from build123d import *

# Parameters (mm, degrees)
SKETCH1_W           = 73
SKETCH1_H           = 20
BOSS_EXTRUDE1_DEPTH = 40
CUT_EXTRUDE1_DEPTH  = 20
FILLET1_R           = 20
FILLET2_R           = 20


with BuildPart() as part:
    # Sketch1 → Boss-Extrude1 (new body)
    with BuildSketch(Plane(origin=(0, 0, 0), x_dir=(1, 0, 0), z_dir=(0, 1, 0))):
        Rectangle(SKETCH1_W, SKETCH1_H)
    extrude(amount=BOSS_EXTRUDE1_DEPTH)

    # Sketch2 → Cut-Extrude1 (cut)
    with BuildSketch(Plane.XY.offset(10)):
        with BuildLine():
            Line((-29, 0), (-29, 2.352421437))
            ThreePointArc((-29, 2.352421437), (-29.878679656, 4.473741781), (-32, 5.352421437))
            Line((-32, 5.352421437), (-33, 5.352421437))
            ThreePointArc((-33, 5.352421437), (-33.707106781, 5.645314656), (-34, 6.352421437))
            Line((-34, 6.352421437), (-34, 9.352421437))
            ThreePointArc((-34, 9.352421437), (-33.707106781, 10.059528218), (-33, 10.352421437))
            Line((-33, 10.352421437), (-31, 10.352421437))
            Line((-31, 10.352421437), (-28, 10.352421437))
            ThreePointArc((-28, 10.352421437), (-25.171572875, 11.523994313), (-24, 14.352421437))
            Line((-24, 14.352421437), (-24, 37))
            Line((-24, 37), (24, 37))
            Line((24, 37), (24, 14.352421437))
            ThreePointArc((24, 14.352421437), (25.171572875, 11.523994313), (28, 10.352421437))
            Line((28, 10.352421437), (31, 10.352421437))
            Line((31, 10.352421437), (33, 10.352421437))
            ThreePointArc((33, 10.352421437), (33.707106781, 10.059528218), (34, 9.352421437))
            Line((34, 9.352421437), (34, 6.352421437))
            ThreePointArc((34, 6.352421437), (33.707106781, 5.645314656), (33, 5.352421437))
            Line((33, 5.352421437), (32, 5.352421437))
            ThreePointArc((32, 5.352421437), (29.878679656, 4.473741781), (29, 2.352421437))
            Line((29, 2.352421437), (29, 0))
            Line((29, 0), (-29, 0))
        make_face()
    extrude(amount=-CUT_EXTRUDE1_DEPTH, mode=Mode.SUBTRACT)

    # Fillet1
    fillet1_edges = [part.edges().sort_by_distance(p)[0] for p in [
        (36.5, 40, 0),
        (-36.5, 40, 0),
    ]]
    fillet(fillet1_edges, radius=FILLET1_R)

    # Fillet2
    fillet2_edges = [part.edges().sort_by_distance(p)[0] for p in [
        (-24, 37, 0),
        (24, 37, 0),
    ]]
    fillet(fillet2_edges, radius=FILLET2_R)


solid = part.part
Check sheet for the modelled part. Datum: model origin and axes. Units: mm. A direction names the side the tool comes from. Coordinates: 2 decimals unless noted, no trailing zeros. Write each loop counter-clockwise with the first axis right and the second up, starting at its lowest first coordinate (ties: lowest second). Pieces come first, ordered by that corner, then holes.
Item 1: Depth check by flat-ended pin: pin 1 Ø6 at (y, z) = (30, 1) entering from +X (3 decimals); pin 2 Ø5 at (x, z) = (-11, 1.5) entering from -Y; pin 3 Ø1 at (x, z) = (-11.5, 4.5) entering from -Y; pin 4 Ø2.5 at (x, z) = (-30.5, -3.5) entering from -Y. Enter the tip coordinate at first touch or a pass-through.
Numbers:
pin 1: stops at x = 35.235
pin 2: stops at y = 34.6
pin 3: stops at y = 35.33
pin 4: stops at y = 0
Item 2: Cross-section at D-D on y = 11.5. Record the boundary of the cut face in (x, z), then the cut area to 3 significant figures.
Numbers:
outline: (-36.5, -10) - (-25.2, -10) - (-25.2, 10) - (-36.5, 10) - close; (25.2, -10) - (36.5, -10) - (36.5, 10) - (25.2, 10) - close
area: 452 mm2
Item 3: Cross-section at C-C on x = -1. Record the boundary of the cut face in (y, z).
Numbers:
outline: (37, -10) - (40, -10) - (40, 10) - (37, 10) - close
Item 4: Scan lines: probe 1 along Y at (x, z) = (-32.5, -0.75); probe 2 along X at (y, z) = (15, 8.5); probe 3 along X at (y, z) = (6.5, -6.5). Record each from-to range of solid material in increasing order.
Numbers:
probe 1: y = 0 to 5.35, 10.35 to 32
probe 2: x = -36.5 to -24, 24 to 36.5
probe 3: x = -36.5 to -34, 34 to 36.5
Item 5: Cross-section at A-A on z = 6.5. Record the boundary of the cut face in (x, y).
Numbers:
outline: (-36.5, 0) - (-29, 0) - (-29, 2.35) arc R3 ccw to (-32, 5.35) - (-33, 5.35) arc R1 cw to (-34, 6.35) - (-34, 9.35) arc R1 cw to (-33, 10.35) - (-28, 10.35) arc R4 ccw to (-24, 14.35) - (-24, 17) arc R20 cw to (-4, 37) - (4, 37) arc R20 cw to (24, 17) - (24, 14.35) arc R4 ccw to (28, 10.35) - (33, 10.35) arc R1 cw to (34, 9.35) - (34, 6.35) arc R1 cw to (33, 5.35) - (32, 5.35) arc R3 ccw to (29, 2.35) - (29, 0) - (36.5, 0) - (36.5, 20) arc R20 ccw to (16.5, 40) - (-16.5, 40) arc R20 ccw to (-36.5, 20) - close
Item 6: Cross-section at B-B on y = 22. Record the boundary of the cut face in (x, z), then the cut area to 3 significant figures.
Numbers:
outline: (-36.4, -10) - (-23.36, -10) - (-23.36, 10) - (-36.4, 10) - close; (23.36, -10) - (36.4, -10) - (36.4, 10) - (23.36, 10) - close
area: 521 mm2
Item 7: Access from +Z, -Z, +X, -X, +Y, -Y to the whole of each face (thin tool, end or side, straight path). Record for faces 1 (the face through (25.1, 11.6, 0.1)), 2 (the face through (-36.5, 10, 0)), 3 (the face through (30, 10.352, 0)).
Numbers:
face 1: +Z, -Z, -Y
face 2: +Z, -Z, -X, +Y, -Y
face 3: +Z, -Z
